Geometry check sheet. Reference: the model listing, model coordinates, mm. Face numbers are marked on the shaded views. A direction names the side the tool comes from. Give positions to 0.01 mm unless a question says otherwise; leave off trailing zeros. Loops run counter-clockwise (first coordinate to the right, second up) from the corner with the lowest first, then second, coordinate; pieces in that order, holes last. Notation, with made-up numbers: (-21.5, 84) - (-0.5, 84) arc R5 ccw to (-0.5, 88) - close; hole circle Ø2 at (-3, 83.25). An arc over 180 degrees is marked (long way). Use a Markdown table: item, result. Add a question column.
1. Material ranges on L1, parallel to X at y = 4.5, z = 8.5; L2, parallel to Y at x = 62.9, z = 1.95; L3, parallel to Y at x = 58.5, z = 0.5, recorded low to high.
2. Cross-section at B-B on x = 47. Enter the section's corners in (y, z).
3. Cross-section at C-C on z = 11.5. Enter the section's corners in (x, y).
4. Cross-section at A-A on x = 62.9. Enter the section's corners in (y, z).
5. Cross-section at D-D on y = -8. Enter the section's corners in (x, z).
6. Draft check along X on the marked faces 1, 2 and 3. Enter one of: pulls with the +X half, pulls with the -X half, needs draft (parallel to the pull), parting line crosses it, or undercut.
7. Set-up check for the marked faces 4 and 5: record each of +Z, -Z, +X, -X, +Y, -Y from which the full face is reachable in a straight line by a thin tool's end or side.
8. Depth check by flat-ended pin: P1, Ø1, axis at x = 26, y = -29.5, coming from the +Z side; P2, Ø6, axis at y = -35, z = 8.5, coming from the +X side; P3, Ø8, axis at x = 35.5, z = 10, coming from the +Y side; P4, Ø4, axis at x = 62.9, y = 7.72, coming from the +Z side. Enter the tip coordinate at first touch or a pass-through.
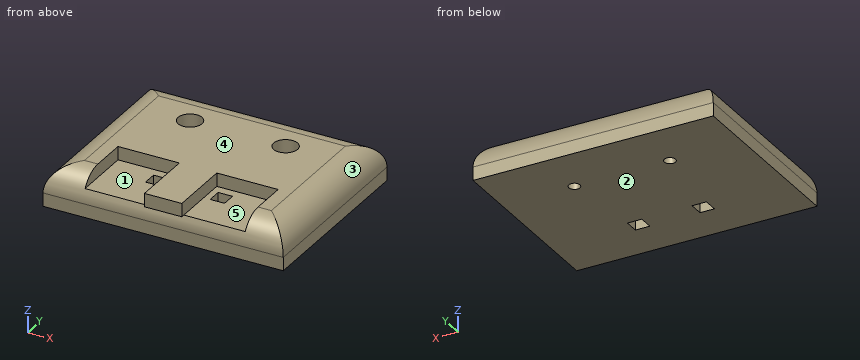
from build123d import *

# Parameters (mm, degrees)
BOSS_EXTRUDE3_DEPTH       = 90
SKETCH3_R                 = 2.1
CUT_EXTRUDE1_DEPTH        = 101.729866263
SKETCH7_W                 = 60
SKETCH7_H                 = 23.583098141
CUT_EXTRUDE3_DEPTH        = 5
SKETCH8_W                 = 5.4
SKETCH8_H                 = 5.4
CUT_EXTRUDE4_DEPTH        = 10.2
FILLET3_R                 = 10
SKETCH9_W                 = 14
SKETCH9_H                 = 23.583098141
BOSS_EXTRUDE4_DEPTH       = 5
ADVANCEDHOLE2_START       = 3.782223439
ADVANCEDHOLE2_OUTLINE_R   = 4.5
ADVANCEDHOLE2_OUTLINE_R_2 = 2.1
ADVANCEDHOLE2_DEPTH       = 10.5


# Read off the part's stored shape, not the designer's step: AdvancedHole2
with BuildPart() as part:
    # Sketch1 → Boss-Extrude3 (new body)
    with BuildSketch(Plane.YZ):
        Polygon((-42.679104458, 14.282223439), (-12.679104458, 14.282223439), (27.320895542, 14.282223439), (27.320895542, -0.717776561), (-42.679104458, -0.717776561), (-42.679104458, 2.342667118), align=None)
    extrude(amount=BOSS_EXTRUDE3_DEPTH)

    # Sketch3 → Cut-Extrude1 (cut, through all)
    with BuildSketch(Plane(origin=(0, 0, -0.717776561), x_dir=(1, 0, 0), z_dir=(0, 0, -1))):
        with Locations(Location((57.1, 25.179104458, 0), (0, 0, 180))):
            Circle(SKETCH3_R)
        with Locations((32.9, 25.179104458)):
            Circle(SKETCH3_R)
        with Locations(Location((62.9, -7.720895542, 0), (0, 0, 180))):
            Circle(SKETCH3_R)
        with Locations((27.1, -7.720895542)):
            Circle(SKETCH3_R)
    extrude(amount=-CUT_EXTRUDE1_DEPTH, mode=Mode.SUBTRACT)

    # Sketch7 → Cut-Extrude3 (cut)
    with BuildSketch(Plane.XY.offset(14.282223439)):
        with Locations((45, -30.887555388)):
            Rectangle(SKETCH7_W, SKETCH7_H)
    extrude(amount=-CUT_EXTRUDE3_DEPTH, mode=Mode.SUBTRACT)

    # Sketch8 → Cut-Extrude4 (cut)
    with BuildSketch(Plane.XY.offset(9.282223439)):
        with Locations((32.9, -25.179104458)):
            Rectangle(SKETCH8_W, SKETCH8_H)
        with Locations((57.1, -25.179104458)):
            Rectangle(SKETCH8_W, SKETCH8_H)
    extrude(amount=-CUT_EXTRUDE4_DEPTH, mode=Mode.SUBTRACT)

    # Fillet3
    # the kernel refuses this fillet: 10 mm, written as the material it takes off along each edge
    with BuildSketch(Plane(origin=(-60, 27.320895542, 14.282223439), x_dir=(0, -1, 0), z_dir=(1, 0, 0))) as fillet3_piece_1:
        with BuildLine():
            CenterArc((FILLET3_R, FILLET3_R), FILLET3_R, 180, 90)
            Line((0, FILLET3_R), (-FILLET3_R * 0.02, FILLET3_R))
            Line((-FILLET3_R * 0.02, FILLET3_R), (-FILLET3_R * 0.02, -FILLET3_R * 0.02))
            Line((-FILLET3_R * 0.02, -FILLET3_R * 0.02), (FILLET3_R, -FILLET3_R * 0.02))
            Line((FILLET3_R, -FILLET3_R * 0.02), (FILLET3_R, 0))
        make_face()
    extrude(amount=210, mode=Mode.SUBTRACT)
    with BuildSketch(Plane(origin=(15, -42.679104458, 14.282223439), x_dir=(0, 1, 0), z_dir=(1, 0, 0)), Plane(origin=(-60, -42.679104458, 14.282223439), x_dir=(0, 1, 0), z_dir=(1, 0, 0))) as fillet3_piece_2:
        with BuildLine():
            CenterArc((FILLET3_R, -FILLET3_R), FILLET3_R, 90, 90)
            Line((0, -FILLET3_R), (-FILLET3_R * 0.0200000000001, -FILLET3_R))
            Line((-FILLET3_R * 0.0200000000001, -FILLET3_R), (-FILLET3_R * 0.02, FILLET3_R * 0.02))
            Line((-FILLET3_R * 0.02, FILLET3_R * 0.02), (FILLET3_R, FILLET3_R * 0.02))
            Line((FILLET3_R, FILLET3_R * 0.02), (FILLET3_R, 0))
        make_face()
    extrude(amount=135, mode=Mode.SUBTRACT)
    with BuildSketch(Plane(origin=(90, -102.679104458, 14.282223439), x_dir=(-1, 0, 0), z_dir=(0, 1, 0)), Plane(origin=(0, 87.320895542, 14.282223439), x_dir=(1, 0, 0), z_dir=(0, -1, 0))) as fillet3_piece_3:
        with BuildLine():
            CenterArc((FILLET3_R, -FILLET3_R), FILLET3_R, 90, 90)
            Line((0, -FILLET3_R), (-FILLET3_R * 0.02, -FILLET3_R))
            Line((-FILLET3_R * 0.02, -FILLET3_R), (-FILLET3_R * 0.02, FILLET3_R * 0.02))
            Line((-FILLET3_R * 0.02, FILLET3_R * 0.02), (FILLET3_R, FILLET3_R * 0.02))
            Line((FILLET3_R, FILLET3_R * 0.02), (FILLET3_R, 0))
        make_face()
    extrude(amount=190, mode=Mode.SUBTRACT)

    # Sketch9 → Boss-Extrude4 (add)
    with BuildSketch(Plane.XY.offset(9.282223439)):
        with Locations((45, -30.887555388)):
            Rectangle(SKETCH9_W, SKETCH9_H)
    extrude(amount=BOSS_EXTRUDE4_DEPTH)

    # AdvancedHole2 outline → AdvancedHole2 (cut)
    # profile 1 of 2: a face of its own
    with BuildSketch(Plane.XY.offset(ADVANCEDHOLE2_START)):
        with Locations((62.9, 7.720895542)):
            Circle(ADVANCEDHOLE2_OUTLINE_R)
        with Locations((62.9, 7.720895542)):
            Circle(ADVANCEDHOLE2_OUTLINE_R_2, mode=Mode.SUBTRACT)
    # profile 2 of 2: a face of its own
    with BuildSketch(Plane.XY.offset(ADVANCEDHOLE2_START)):
        with Locations((27.1, 7.720895542)):
            Circle(ADVANCEDHOLE2_OUTLINE_R)
        with Locations((27.1, 7.720895542)):
            Circle(ADVANCEDHOLE2_OUTLINE_R_2, mode=Mode.SUBTRACT)
    extrude(amount=ADVANCEDHOLE2_DEPTH, mode=Mode.SUBTRACT)


solid = part.part
Values found:
| question | item | result |
|---|---|---|
| 1 | L1 | x = 0.93 to 23.96, 30.24 to 59.76, 66.04 to 89.07 |
| 1 | L2 | y = -42.68 to 5.62, 9.82 to 27.32 |
| 1 | L3 | y = -42.68 to -27.88, -22.48 to 27.32 |
| 2 | outline | (-42.68, -0.72) - (27.32, -0.72) - (27.32, 4.28) arc R10 ccw to (17.32, 14.28) - (-42.68, 14.28) - (-42.68, 9.28) - (-41.34, 9.28) arc R10 ccw to (-42.68, 4.28) - close |
| 3 | outline | (3.08, -39.6) - (15, -39.6) - (15, -19.1) - (38, -19.1) - (38, -42.68) - (52, -42.68) - (52, -19.1) - (75, -19.1) - (75, -39.6) - (86.92, -39.6) - (86.92, 24.24) - (3.08, 24.24) - close; hole circle Ø9 at (27.1, 7.72); hole circle Ø9 at (62.9, 7.72) |
| 4 | outline | (-42.68, -0.72) - (5.62, -0.72) - (5.62, 3.78) - (3.22, 3.78) - (3.22, 14.28) - (-19.1, 14.28) - (-19.1, 9.28) - (-41.34, 9.28) arc R10 ccw to (-42.68, 4.28) - close; (9.82, -0.72) - (27.32, -0.72) - (27.32, 4.28) arc R10 ccw to (17.32, 14.28) - (12.22, 14.28) - (12.22, 3.78) - (9.82, 3.78) - close |
| 5 | outline | (0, -0.72) - (90, -0.72) - (90, 4.28) arc R10 ccw to (80, 14.28) - (10, 14.28) arc R10 ccw to (0, 4.28) - close |
| 6 | face 1 | undercut |
| 6 | face 2 | needs draft |
| 6 | face 3 | pulls with the +X half |
| 7 | face 4 | +Z, +X, -X, +Y, -Y |
| 7 | face 5 | +Z, -Y |
| 8 | P1 | stops at z = 9.28 |
| 8 | P2 | stops at x = 89.93 |
| 8 | P3 | stops at y = 27.17 |
| 8 | P4 | passes through |
